Check sheet for the modelled part. Datum: model origin and axes. Units: mm. Face numbers are marked on the shaded views. A direction names the side the tool comes from. Coordinates: 2 decimals unless noted, no trailing zeros. Order: outer loops, then holes, each group sorted by start corner. A loop starts at its lowest first (then second) coordinate and runs counter-clockwise, first axis right, second up. Notation, with made-up numbers: (57.5, -13.5) -> (114.5, -13.5) arc R14 cw to (114.5, -1.5) -> close; hole circle Ø9 at (22.25, -29). An arc over 180 degrees is marked (long way). Put each result on its own line as item: value. Start each with the question number.
```python
from build123d import *

# Parameters (mm, degrees)
SKETCH1_R               = 20
SKETCH1_R_2             = 14
BOSS_EXTRUDE1_DEPTH     = 30
SKETCH3_W               = 17
SKETCH3_H               = 4.747307011
SKETCH4_W               = 100
SKETCH4_H               = 50
SKETCH4_R               = 14
BOSS_EXTRUDE2_DEPTH     = 15
CUT_EXTRUDE2_DEPTH      = 64.442887702
CUT_EXTRUDE2_DEPTH_BACK = 64.442887702
SKETCH5_W               = 7
SKETCH5_H               = 15


with BuildPart() as part:
    # Sketch1 → Boss-Extrude1 (new body)
    with BuildSketch(Plane(origin=(0, 0, 0), x_dir=(1, 0, 0), z_dir=(0, 1, 0))):
        with Locations(Location((0, 0, 0), (0, 0, 270))):
            Circle(SKETCH1_R)
        with Locations(Location((0, 0, 0), (0, 0, 270))):
            Circle(SKETCH1_R_2, mode=Mode.SUBTRACT)
    extrude(amount=BOSS_EXTRUDE1_DEPTH)

    # Sketch3 → Cut-Revolve2 (revolve, cut)
    with BuildSketch(Plane.XY, mode=Mode.PRIVATE) as cut_revolve2_sk:
        Polygon((-17, 30), (-0.03686902, 19.405086722), (0, 30), align=None)
        with Locations((-8.5, 32.373653506)):
            Rectangle(SKETCH3_W, SKETCH3_H)
    revolve(cut_revolve2_sk.sketch.rotate(Axis((0, 34.747307011, 0), (0, -1, 0)), 270), axis=Axis((0, 34.747307011, 0), (0, -1, 0)), mode=Mode.SUBTRACT)

    # Sketch4 → Boss-Extrude2 (add)
    with BuildSketch(Plane(origin=(0, 0, 0), x_dir=(1, 0, 0), z_dir=(0, 1, 0))):
        Rectangle(SKETCH4_W, SKETCH4_H)
        with Locations(Location((0, 0, 0), (0, 0, 270))):
            Circle(SKETCH4_R, mode=Mode.SUBTRACT)
    extrude(amount=BOSS_EXTRUDE2_DEPTH)

    # Sketch5 → Cut-Extrude2 (cut, two sides: drawn at the far end of the back side and taken through both)
    with BuildSketch(Plane.XY.offset(-CUT_EXTRUDE2_DEPTH_BACK)):
        with Locations((-42.5, 0)):
            Rectangle(SKETCH5_W, SKETCH5_H)
        with Locations((42.5, 0)):
            Rectangle(SKETCH5_W, SKETCH5_H)
    extrude(amount=CUT_EXTRUDE2_DEPTH + CUT_EXTRUDE2_DEPTH_BACK, mode=Mode.SUBTRACT)


solid = part.part
```
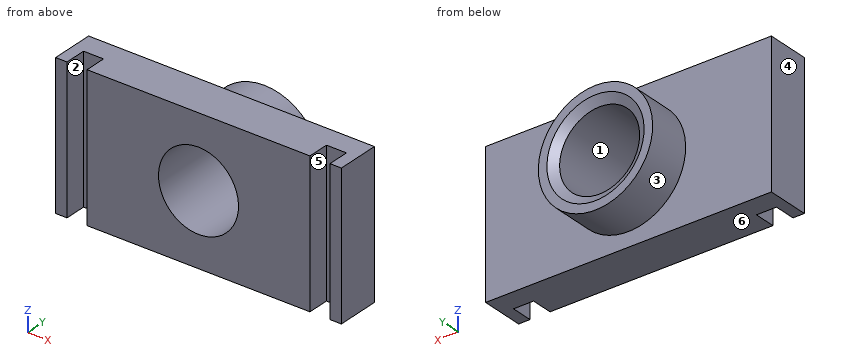
1) Mould release check, pull along X, two halves, no side actions. Record for the marked faces 4, 5 and 6: +X half, -X half, draft (parallel to the pull), parting line (faces both ways), or undercut.
2) Access from +Z, -Z, +X, -X, +Y, -Y to the whole of each face (thin tool, end or side, straight path). Record for the marked faces 1, 2 and 3.
3) Sectioned sample at C-C (z = 0). Record the boundary of the cut face in (x, y), plus the area to 3 significant figures.
4) Scan lines: line 1 along X through (y, z) = (13, 0); line 2 along X through (y, z) = (21, 0); line 3 along Y through (x, z) = (36, -10). Record each from-to range of solid material in increasing order. Write a range as [from, to].
5) Gauge pin test, flat ends, axial feed: pin 1 (4 mm diameter, centred on x = -26, z = 17.5, fed in from +Y); pin 2 (3.5 mm diameter, centred on x = -41.5, z = -3.5, fed in from -Y); pin 3 (10 mm diameter, centred on x = -4.5, y = 27, fed in from -Z). Record the tip position at first contact, or that the pin passes through.
6) Sectioned sample at A-A (y = 4). Record the boundary of the cut face in (x, z), plus the area to 3 significant figures.
7) Sectioned sample at D-D (y = 9). Record the boundary of the cut face in (x, z).
8) Sectioned sample at B-B (x = 0). Record the boundary of the cut face in (y, z).
Entries:
1. face 4: -X half
1. face 5: undercut
1. face 6: draft
2. face 1: +Y, -Y
2. face 2: +Z, -Z, -Y
2. face 3: +Y
3. outline: (-50, 0) -> (-46, 0) -> (-46, 7.5) -> (-39, 7.5) -> (-39, 0) -> (-14, 0) -> (-14, 28.13) -> (-17, 30) -> (-20, 30) -> (-20, 15) -> (-50, 15) -> close; (14, 0) -> (39, 0) -> (39, 7.5) -> (46, 7.5) -> (46, 0) -> (50, 0) -> (50, 15) -> (20, 15) -> (20, 30) -> (17, 30) -> (14, 28.13) -> close
3. area: 1,150 mm2
4. line 1: x = [-50, -14], [14, 50]
4. line 2: x = [-20, -14], [14, 20]
4. line 3: y = [0, 15]
5. pin 1: stops at y = 15
5. pin 2: stops at y = 7.5
5. pin 3: stops at z = -20
6. outline: (-50, -25) -> (-46, -25) -> (-46, 25) -> (-50, 25) -> close; (-39, -25) -> (39, -25) -> (39, 25) -> (-39, 25) -> close; (46, -25) -> (50, -25) -> (50, 25) -> (46, 25) -> close; hole circle Ø28 at (0, 0)
6. area: 3,680 mm2
7. outline: (-50, -25) -> (50, -25) -> (50, 25) -> (-50, 25) -> close; hole circle Ø28 at (0, 0)
8. outline: (0, -25) -> (15, -25) -> (15, -20) -> (30, -20) -> (30, -17) -> (28.13, -14) -> (0, -14) -> close; (0, 14) -> (28.13, 14) -> (30, 17) -> (30, 20) -> (15, 20) -> (15, 25) -> (0, 25) -> close
